Read the model definition and answer for the solid it produces. Units are mm, in the model's axes. Coordinates: 2 decimals unless noted, no trailing zeros. Write each loop counter-clockwise with the first axis right and the second up, starting at its lowest first coordinate (ties: lowest second). Pieces come first, ordered by that corner, then holes. Notation, with made-up numbers: (10, 16.25) -> (45, 16.25) arc R28 cw to (45, 48.25) -> close; hole circle Ø7 at (5.5, -37). An arc over 180 degrees is marked (long way). Answer as a JSON object with one key per item and string values. Group by question number.
(1) Straight lines are drawn through the part: L1, parallel to X at y = 15.5, z = 287; L2, parallel to Y at x = 5.75, z = 316; L3, parallel to Y at x = -6.5, z = 225. For each, find the intervals that lie inside material, in ascending order.
(2) Find section A-A (z = 334). Give the vertices of the cut face in (x, y), then the cut area to 3 significant figures.
(3) Find section C-C (x = 2). Give the vertices of the cut face in (y, z).
(4) Flat-ended cylindrical pins translate along their axes: P1, Ø10, axis at x = 3.5, y = 15.5, coming from the -Z side; P2, Ø1.5, axis at x = 7, z = 157, coming from the -Y side. Find the tip coordinate at first contact, or state that the pin passes through.
Autodesk Inventor part; units mm, degrees
ref_plane "Start Plane" through (0, 0, -6.6189) normal (0, 0, 1) x (1, 0, 0)
ref_plane "End Plane" through (0, 0, 608.6348) normal (0, 0, 1) x (1, 0, 0)
ref_plane "Work Plane4" through (-342.9253, 16, 828.9932) normal (0.5519, 0, 0.8339) x (0.8339, 0, -0.5519)
ref_plane "Start Plane" through (0, 0, -6.6189) normal (0, 0, 1) x (1, 0, 0)
ref_plane "End Plane" through (0, 0, 608.6348) normal (0, 0, 1) x (1, 0, 0)
sketch "Sketch" plane through (0, 0, 0) normal (0, 0, 1) x (1, 0, 0)
  line L0 (-10, -16) -> (-10, 16)
  line L1 (-6, 20) -> (6, 20)
  line L2 (10, 16) -> (10, -16)
  line L3 (6, -20) -> (-6, -20)
  arc A0 (-10, -16) -> (-6, -20) centre (-6, -16) ccw
  arc A1 (10, 16) -> (6, 20) centre (6, 16) ccw
  arc A2 (-6, 20) -> (-10, 16) centre (-6, 16) ccw
  arc A3 (6, -20) -> (10, -16) centre (6, -16) ccw
  arc A4 (-6, 18) -> (-8, 16) centre (-6, 16) ccw
  line L4 (-6, 18) -> (6, 18)
  arc A5 (8, 16) -> (6, 18) centre (6, 16) ccw
  line L5 (8, 16) -> (8, -16)
  arc A6 (6, -18) -> (8, -16) centre (6, -16) ccw
  line L6 (6, -18) -> (-6, -18)
  arc A7 (-8, -16) -> (-6, -18) centre (-6, -16) ccw
  line L7 (-8, -16) -> (-8, 16)
  line L8 (0, 29.1598) -> (0, -29.1598) construction
  line L9 (-15.1598, 0) -> (15.1598, 0) construction
  dimension "d7" = 4
  dimension "d9" = 20
  dimension "d11" = 40
  dimension "d12" = 2
  dimension "d15" = 10
  dimension "d16" = 20
extrude "Body" add sketch "Sketch" along normal up to surface (615.2536 mm away) from surface at -6.6189
sketch "Sketch3" plane through (0, 0, 0) normal (0, 0, 1) x (1, 0, 0)
  line L0 (0, 0) -> (10, 0)
ref_plane "Work Plane3" through (0, 0, 0) normal (0, -1, 0) x (1, 0, 0)
ref_plane "Work Plane4" through (-342.9253, 16, 828.9932) normal (0.5519, 0, 0.8339) x (0.8339, 0, -0.5519)
split "Split1" plane through (-342.9253, 16, 828.9932) removes the side toward (0.5519, 0, 0.8339)
ref_plane "Work Plane5" through (-331.8866, -16, 219.6709) normal (-0.5519, 0, -0.8339) x (-0.8339, 0, 0.5519)
split "Split2" plane through (-331.8866, -16, 219.6709) removes the side toward (-0.5519, 0, -0.8339)
sketch "Sketch4" plane through (0, 0, 0) normal (0, -1, 0) x (1, 0, 0)
  line L0 (-2, -6.6189) -> (12, -6.6189)
  line L1 (-2, 608.6348) -> (12, 608.6348)
  dimension "d18" = 615.2536
equation "\"d7\" = G_IR"
equation "\"d9\" = G_W"
equation "\"d11\" = G_H"
equation "\"d12\" = G_T"
equation "\"d15\" = 0.5 * d9"
equation "\"d16\" = 0.5 * d11"
equation "\"d3\" = G_L"
equation "\"G_W\" = 20"
equation "\"G_H\" = 40"
equation "\"G_T\" = 2"
equation "\"G_IR\" = 4"
equation "\"G_L\" = d18"
equation "\"G_OFFSET_START\" = 6.61886"
equation "\"G_OFFSET_END\" = -17.36524"
equation "\"d13\" = -G_OFFSET_START"
equation "\"d14\" = G_OFFSET_END + B_L"
equation "\"B_L\" = 626"
properties part number "ISO 4019 - 40x20x2 - 615,25" material "Steel, Mild"
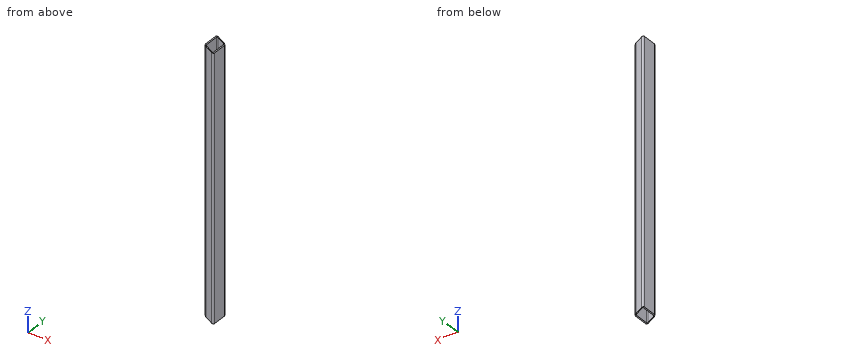
Results below:
{
 "1": {"L1": "x = -10 to -8, 8 to 10", "L2": "y = -20 to -18, 18 to 20", "L3": "y = -19.97 to -17.94, 17.94 to 19.97"},
 "2": {"outline": "(-10, -16) arc R4 ccw to (-6, -20) -> (6, -20) arc R4 ccw to (10, -16) -> (10, 16) arc R4 ccw to (6, 20) -> (-6, 20) arc R4 ccw to (-10, 16) -> close; hole (-8, -16) arc R2 ccw to (-6, -18) -> (6, -18) arc R2 ccw to (8, -16) -> (8, 16) arc R2 ccw to (6, 18) -> (-6, 18) arc R2 ccw to (-8, 16) -> close", "area": "214 mm2"},
 "3": {"outline": "(-20, -1.32) -> (-18, -1.32) -> (-18, 600.69) -> (-20, 600.69) -> close; (18, -1.32) -> (20, -1.32) -> (20, 600.69) -> (18, 600.69) -> close"},
 "4": {"P1": "stops at z = -5.63", "P2": "stops at y = -19.99"}
}
